Read the model definition and answer for the solid it produces. Units are mm, in the model's axes. Face numbers are marked on the shaded views. A direction names the side the tool comes from. Coordinates: 2 decimals unless noted, no trailing zeros. Order: outer loops, then holes, each group sorted by start corner. A loop starts at its lowest first (then second) coordinate and runs counter-clockwise, first axis right, second up.
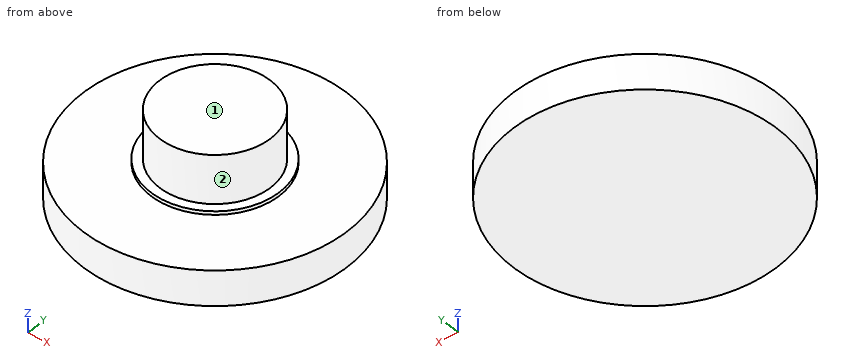
```python
from build123d import *

# Parameters (mm, degrees)
F0_R     = 9.525
F0_R_2   = 4.635
F1_DEPTH = 2.54
F0_R_3   = 4
F2_DEPTH = 2.794
F3_DEPTH = 6.294


with BuildPart() as f1:
    # F0 (on Top) → F1 (new body)
    with BuildSketch(Plane.XY):
        with Locations((-69.424219, 31.217609)):
            Circle(F0_R)
        with Locations((-69.424219, 31.217609)):
            Circle(F0_R_2, mode=Mode.SUBTRACT)
    extrude(amount=F1_DEPTH)

    # F0 (on Top) → F2 (join)
    with BuildSketch(Plane.XY):
        with Locations((-69.424219, 31.217609)):
            Circle(F0_R_2)
        with Locations((-69.424219, 31.217609)):
            Circle(F0_R_3, mode=Mode.SUBTRACT)
    extrude(amount=F2_DEPTH)

    # F0 (on Top) → F3 (join)
    with BuildSketch(Plane.XY):
        with Locations((-69.424219, 31.217609)):
            Circle(F0_R_3)
    extrude(amount=F3_DEPTH)


solid = f1.part
```
1) A cutting plane is placed at C-C, the plane z = 4.75. Determine the outline of the cut face in (x, y), and give its area (3 significant figures).
A:
outline: circle Ø8 at (-69.42, 31.22)
area: 50.3 mm2
2) Flat-ended cylindrical pins translate along their axes: pin 1 Ø3 at (x, z) = (-74.5, 3.5) entering from -Y; pin 2 Ø5.5 at (x, y) = (-69.5, 27) entering from +Z; pin 3 Ø1 at (x, z) = (-71, 2) entering from +Y; pin 4 Ø3 at (x, z) = (-74, 3.5) entering from -Y. Find the tip coordinate at first contact, or state that the pin passes through.
A:
pin 1: stops at y = 22.54
pin 2: stops at z = 6.29
pin 3: stops at y = 40.68
pin 4: stops at y = 22.33
3) A cutting plane is placed at B-B, the plane y = 33.75. Determine the outline of the cut face in (x, z), and give its area (3 significant figures).
A:
outline: (-78.61, 0) - (-60.24, 0) - (-60.24, 2.54) - (-65.54, 2.54) - (-65.54, 2.79) - (-66.33, 2.79) - (-66.33, 6.29) - (-72.52, 6.29) - (-72.52, 2.79) - (-73.31, 2.79) - (-73.31, 2.54) - (-78.61, 2.54) - close
area: 70.3 mm2
4) Straight lines are drawn through the part: line 1 (Z direction, x = -76.25, y = 29.25); line 2 (X direction, y = 31.25, z = 4); line 3 (X direction, y = 28.5, z = 1). For each, find the intervals that lie inside material, in ascending order.
A:
line 1: z = 0 to 2.54
line 2: x = -73.42 to -65.42
line 3: x = -78.55 to -60.3
5) A cutting plane is placed at A-A, the plane x = -67.25. Determine the outline of the cut face in (y, z), and give its area (3 significant figures).
A:
outline: (21.94, 0) - (40.49, 0) - (40.49, 2.54) - (35.31, 2.54) - (35.31, 2.79) - (34.58, 2.79) - (34.58, 6.29) - (27.86, 6.29) - (27.86, 2.79) - (27.12, 2.79) - (27.12, 2.54) - (21.94, 2.54) - close
area: 72.7 mm2
6) Which of the six approach directions +Z, -Z, +X, -X, +Y, -Y give full straight-line access (tool end or side, diameter ignored) to the marked faces 1 and 2?
A:
face 1: +Z, +X, -X, +Y, -Y
face 2: +Z
7) A cutting plane is placed at D-D, the plane x = -64. Determine the outline of the cut face in (y, z), and give its area (3 significant figures).
A:
outline: (23.39, 0) - (39.05, 0) - (39.05, 2.54) - (23.39, 2.54) - close
area: 39.8 mm2
